Work out the finished part from the listing and answer in its coordinate system (mm). Face numbers are marked on the shaded views. A direction names the side the tool comes from. Round coordinates to 2 decimals unless told otherwise and drop trailing zeros. Write each loop counter-clockwise with the first axis right and the second up, starting at its lowest first coordinate (ties: lowest second). Pieces come first, ordered by that corner, then holes. Notation, with made-up numbers: M -40,37 L 4,37 A35 cw 4,70 Z; hole C 33.25,-7 d8. An arc over 180 degrees is marked long. One line per item, written item: value. Start each with the question number.
Q1. Find section C-C (x = 6.5). Write down the section's boundary in (y, z), and give its area (3 significant figures).
Q2. Find section D-D (z = 2). Write down the section's boundary in (x, y), and give its area (3 significant figures).
Q3. A tool of negligible diameter and unlimited length cuts with its end or side. For the marked faces 4 and 5, from which of +Z, -Z, +X, -X, +Y, -Y can it reach the whole face along a straight path? Write none if from no direction.
Q4. Find section A-A (z = 0). Write down the section's boundary in (x, y), and give its area (3 significant figures).
Q5. The mould has two halves that part along Z. Classify the marked faces 1, 2 and 3: released by +Z, released by -Z, zero draft, split by the parting line, or undercut.
Q6. Consider probe 1 along Y at (x, z) = (10.5, 0); probe 2 along Y at (x, z) = (2, 0); probe 3 along X at (y, z) = (-1.5, 2). Determine where each line is inside the solid, lowest interval first.
Q7. Given pin 1 Ø3.5 at (y, z) = (0, 0) entering from -X; pin 2 Ø5 at (x, z) = (4.5, -3.5) entering from -Y; pin 3 Ø5 at (x, y) = (9, 1.5) entering from -Z, each flat-ended and moving along its own axis, determine where each tip first touches the part or whether it passes through.
from build123d import *

# Parameters (mm, degrees)
SKETCH1_R           = 5.8
BOSS_EXTRUDE1_DEPTH = 4
SKETCH2_R           = 4
BOSS_EXTRUDE2_DEPTH = 11.5
SKETCH3_R           = 1.5
CUT_EXTRUDE1_DEPTH  = 20
SKETCH4_R           = 3
CUT_EXTRUDE2_DEPTH  = 3


with BuildPart() as part:
    # Sketch1 → Boss-Extrude1 (new body)
    with BuildSketch(Plane(origin=(0, 0, 0), x_dir=(0, 0, -1), z_dir=(1, 0, 0))):
        Circle(SKETCH1_R)
    extrude(amount=BOSS_EXTRUDE1_DEPTH)

    # Sketch2 → Boss-Extrude2 (add)
    with BuildSketch(Plane(origin=(4, 0, 0), x_dir=(0, 0, -1), z_dir=(1, 0, 0))):
        Circle(SKETCH2_R)
    extrude(amount=BOSS_EXTRUDE2_DEPTH)

    # Sketch3 → Cut-Extrude1 (cut)
    with BuildSketch(Plane.ZY):
        Circle(SKETCH3_R)
    extrude(amount=-CUT_EXTRUDE1_DEPTH, mode=Mode.SUBTRACT)

    # Sketch4 → Cut-Extrude2 (cut)
    with BuildSketch(Plane.ZY):
        Circle(SKETCH4_R)
    extrude(amount=-CUT_EXTRUDE2_DEPTH, mode=Mode.SUBTRACT)


solid = part.part
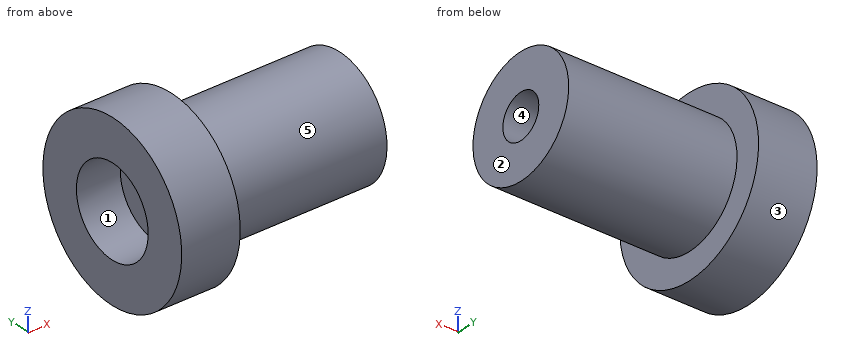
The answers:
1. outline: C 0,0 d8; hole C 0,0 d3
1. area: 43.2 mm2
2. outline: M 0,-5.44 L 4,-5.44 L 4,-3.46 L 15.5,-3.46 L 15.5,3.46 L 4,3.46 L 4,5.44 L 0,5.44 L 0,2.24 L 3,2.24 L 3,-2.24 L 0,-2.24 Z
2. area: 110 mm2
3. face 4: +X, -X
3. face 5: +X
4. outline: M 0,-5.8 L 4,-5.8 L 4,-4 L 15.5,-4 L 15.5,-1.5 L 3,-1.5 L 3,-3 L 0,-3 Z; M 0,3 L 3,3 L 3,1.5 L 15.5,1.5 L 15.5,4 L 4,4 L 4,5.8 L 0,5.8 Z
4. area: 82.9 mm2
5. face 1: undercut
5. face 2: zero draft
5. face 3: split by the parting line
6. probe 1: -4 to -1.5, 1.5 to 4
6. probe 2: -5.8 to -3, 3 to 5.8
6. probe 3: 3 to 15.5
7. pin 1: x = 3
7. pin 2: y = -5.7
7. pin 3: z = -4
